CAD build for the part. Positions are in the model's coordinates, mm. A direction names the side the tool comes from. Give positions to 0.01 mm unless a question says otherwise; leave off trailing zeros. Loops run counter-clockwise (first coordinate to the right, second up) from the corner with the lowest first, then second, coordinate; pieces in that order, holes last. Notation, with made-up numbers: M 74,-30.75 L 114,-30.75 A21 ccw 114,-13.75 Z; hole C 56,52 d7. An arc over 180 degrees is marked long. Answer as CSV lines item,"result".
Autodesk Inventor part; units mm, degrees
ref_plane "Work Plane1" through (30.1625, 0, 0) normal (0, 0, -1) x (1, 0, 0)
ref_plane "YZ Plane" through (0, 0, 0) normal (1, 0, 0) x (0, 1, 0)
ref_plane "XZ Plane" through (0, 0, 0) normal (0, 1, 0) x (-1, 0, 0)
sketch "Sketch1" plane through (0, 0, 0) normal (0, 0, 1) x (1, 0, 0)
  line L0 (-1.8, 0) -> (5, 0)
  line L1 (5, 0) -> (5, 1.5)
  line L2 (5, 1.5) -> (1, 1.5)
  line L3 (1, 1.5) -> (0.6932, 1.1935)
  line L4 (0.6932, 1.1935) -> (0, 1.1935)
  line L5 (0, 1.1935) -> (0, 3)
  line L6 (-3.16, 0) -> (6.36, 0)
  line L7 (0, -0.6) -> (0, 3.6)
  line L8 (-1.8, 0) -> (-1.8, 2.9997)
  line L9 (0, 3) -> (-1.8, 2.9997)
  line L10 (1, 1.5) -> (0, 1.5) construction
  dimension "d0" = 5
  dimension "d1" = 4
  dimension "d2" = 0.3068
  dimension "d3" = 1.8
  dimension "d4" = 3
  dimension "d5" = 2.387
  dimension "d9" = 6
  dimension "d10" = 0.01
revolve "Body" add sketch "Sketch1" angle 360 about axis through (-1.8, 0, 0) along (1, 0, 0)
sketch "Sketch2" plane through (-1.8, 0, 0) normal (-1, 0, 0) x (0, 0, 1)
  circle A0 centre (0, 0) radius 3
  line L0 (0, 0) -> (0, 2.9997)
  line L1 (-3, 0.5) -> (3, 0.5)
  line L2 (3, 0.5) -> (3, -0.5)
  line L3 (3, -0.5) -> (-3, -0.5)
  line L4 (-3, -0.5) -> (-3, 0.5)
  line L5 (-3, 0) -> (3, 0) construction
  line L6 (0, 0.5) -> (0, -0.5) construction
  dimension "d11" = 1
  dimension "d12" = 6
fillet "Fillet1" radius 1.2 1 edges at (-1.8, -2.9997, 0)
extrude "Slot" cut sketch "Sketch2" against normal blind 0.72 contours A0 L3 L1 | L2 L3 A0 | A0 L1 L2 | L3 L4 A0 | A0 L4 L1
thread "Thread"
chamfer "Chamfer1" distance 0.3067 distance2 0.3068 1 edges at (5, -1.5, 0) measured on face at (5, 0.8773, -0.3972)
ref_plane "Work Plane1" through (30.1625, 0, 0) normal (0, 0, -1) x (1, 0, 0)
equation "\"d11\" = SBR"
equation "\"d12\" = KOD"
equation "\"d14\" = RR"
equation "\"d19\" = STI"
equation "\"d15\" = GEL"
equation "\"d17\" = -0.5 * SPD + 0.5 * GD"
equation "\"d0\" = NLG"
equation "\"d1\" = GEL"
equation "\"d3\" = KOH"
equation "\"d4\" = GD"
equation "\"d5\" = BDM"
equation "\"d9\" = KOD"
equation "\"d10\" = KEWI"
equation "\"GD\" = NND"
equation "\"NLG\" = 5"
equation "\"GEL\" = 4"
equation "\"KOD\" = 6"
equation "\"KOH\" = 1.8"
equation "\"GAL\" = 0.61345 * PTC"
equation "\"SPD\" = NND - 1.2269 * PTC"
equation "\"BDM\" = 2.387"
equation "\"GUL\" = 0.61345 * PTC"
equation "\"RR\" = 1.2"
equation "\"SBR\" = 1"
equation "\"STI\" = 0.72"
equation "\"KEWI\" = 0.01deg"
equation "\"PTC\" = 0.5"
equation "\"THREADDIA\" = 3"
equation "\"TOA\" = 30deg"
equation "\"NND\" = 3"
equation "\"RR1\" = 0.3"
equation "\"GD1\" = THREADDIA - 1.2269 * PTC"
properties part number "AS 1427 - M3 x 5" material "Steel, Mild"
Q1. Mould opens along Y. For faces 1 (the cylindrical face through (-0.3, -3, -0.1)), 2 (the flat face through (-1.8, -1, 0)), 3 (the flat face through (-1.08, 0, 0)) say: released by +Y, released by -Y, zero draft, split by the parting line, or undercut.
Solution:
face 1,"split by the parting line"
face 2,"zero draft"
face 3,"undercut"
Q2. Wall check: line 1 (X direction, y = 1.5, z = 0.5); line 2 (X direction, y = 0.75, z = 1.25); line 3 (Z direction, x = -0.5, y = -1.75). Give the ranges that are in metal, low to high. Write a range as [from, to].
Solution:
line 1,"x = [-1.8, 0]"
line 2,"x = [-1.8, 0], [0.96, 4.74]"
line 3,"z = [-2.44, 2.44]"
Q3. Cut at B-B (z = 0). Write the cut outline in (x, y), and give its area (3 significant figures).
Solution:
outline,"M -1.8,-1.8 A1.2 ccw -0.6,-3 L 0,-3 L 0,-1.19 L 0.69,-1.19 L 1,-1.5 L 4.69,-1.5 L 5,-1.19 L 5,1.19 L 4.69,1.5 L 1,1.5 L 0.69,1.19 L 0,1.19 L 0,3 L -0.6,3 A1.2 ccw -1.8,1.8 L -1.8,0.5 L -1.08,0.5 L -1.08,-0.5 L -1.8,-0.5 Z"
area,"23.8 mm²"
Q4. Which spindle directions (+Z, -Z, +X, -X, +Y, -Y) get a long thin tool onto all of the face, cutting with end or side? Do faces 4 (the flat face through (5, 0, 0)), 5 (the cylindrical face through (2.82, -1.5, -0.07)), 6 (the flat face through (0, 1, -1)). Say none if no direction does.
Solution:
face 4,"+Z, -Z, +X, +Y, -Y"
face 5,"+X"
face 6,"none"
Q5. Cut at C-C (x = 0.25). Write the cut outline in (y, z), and give its area (3 significant figures).
Solution:
outline,"C 0,0 d2.39"
area,"4.48 mm²"
Q6. Cut at D-D (x = 3.25). Write the cut outline in (y, z), and give its area (3 significant figures).
Solution:
outline,"C 0,0 d3"
area,"7.07 mm²"
Q7. Cut at A-A (y = 0). Write the cut outline in (x, z).
Solution:
outline,"M -1.08,-2.9 A1.2 ccw -0.6,-3 L 0,-3 L 0,-1.19 L 0.69,-1.19 L 1,-1.5 L 4.69,-1.5 L 5,-1.19 L 5,1.19 L 4.69,1.5 L 1,1.5 L 0.69,1.19 L 0,1.19 L 0,3 L -0.6,3 A1.2 ccw -1.08,2.9 Z"
Q8. Pin check, flat tips, straight feed: P1, Ø0.5, axis at y = 0, z = -0.5, coming from the -X side; P2, Ø3, axis at x = 0.5, z = -0.5, coming from the -Y side; P3, Ø0.6, axis at x = -1.5, z = -1, coming from the -Y side; P4, Ø1.5, axis at x = 3.5, z = 2, coming from the +Y side. Stop position of each tip, or through.
Solution:
P1,"stops at x = -1.08"
P2,"stops at y = -3"
P3,"stops at y = -2.68"
P4,"stops at y = 0.83"
